Input: part model. Units: mm. Frame: model coordinates. A direction names the side the tool comes from. Coordinates: 2 decimals unless noted, no trailing zeros. Write each loop counter-clockwise with the first axis right and the second up, starting at its lowest first coordinate (ties: lowest second). Pieces come first, ordered by that corner, then holes. Notation, with made-up numbers: M 25.25,-28 L 34.25,-28 A30 ccw 34.25,0 Z; hole C -37.75,0 d8. An arc over 180 degrees is marked long. Use one line per item in the form item = value.
from build123d import *

# Parameters (mm, degrees)
SKETCH1_W               = 117.85
SKETCH1_H               = 100
BOSS_EXTRUDE1_DEPTH     = 3
BOSS_EXTRUDE2_DEPTH     = 117.85
SKETCH3_W               = 10
SKETCH3_H               = 24
CUT_EXTRUDE1_DEPTH      = 3
CUT_EXTRUDE2_DEPTH      = 129.579245993
CUT_EXTRUDE2_DEPTH_BACK = 129.579245993
SKETCH4_W               = 11.05
SKETCH4_H               = 9
SKETCH4_W_2             = 84.75
SKETCH5_W               = 92.85
SKETCH5_H               = 3
CUT_EXTRUDE3_DEPTH      = 3


with BuildPart() as part:
    # Sketch1 → Boss-Extrude1 (new body)
    with BuildSketch(Plane(origin=(0, 0, 0), x_dir=(1, 0, 0), z_dir=(0, 1, 0))):
        with Locations((58.925, 50)):
            Rectangle(SKETCH1_W, SKETCH1_H)
    extrude(amount=BOSS_EXTRUDE1_DEPTH)

    # Sketch2 → Boss-Extrude2 (add)
    with BuildSketch(Plane(origin=(117.85, 0, 0), x_dir=(0, 0, -1), z_dir=(1, 0, 0))):
        Polygon((4.2, 6), (4.2, 3), (6.5, 3), (6.5, 12), (4.2, 12), align=None)
        Polygon((4.2, 12), (4.2, 6), (1.2, 8.517298894), align=None)
    boss_extrude2 = extrude(amount=-BOSS_EXTRUDE2_DEPTH)

    # Sketch3 → Cut-Extrude1 (cut)
    with BuildSketch(Plane.XZ):
        with Locations((112.85, -56)):
            Rectangle(SKETCH3_W, SKETCH3_H)
    extrude(amount=-CUT_EXTRUDE1_DEPTH, mode=Mode.SUBTRACT)

    # Mirror1: Boss-Extrude2 across plane
    add(boss_extrude2.mirror(Plane.XY.offset(-50)))

    # Sketch4 → Cut-Extrude2 (cut, two sides: drawn at the far end of the back side and taken through both)
    with BuildSketch(Plane.XY.offset(-50).offset(-CUT_EXTRUDE2_DEPTH_BACK)):
        with Locations((5.525, 7.5)):
            Rectangle(SKETCH4_W, SKETCH4_H)
        with Locations((112.325, 7.5)):
            Rectangle(SKETCH4_W, SKETCH4_H)
        with Locations((58.925, 7.5)):
            Rectangle(SKETCH4_W_2, SKETCH4_H)
    extrude(amount=CUT_EXTRUDE2_DEPTH + CUT_EXTRUDE2_DEPTH_BACK, mode=Mode.SUBTRACT)

    # Sketch5 → Cut-Extrude3 (cut)
    with BuildSketch(Plane(origin=(0, 0, 0), x_dir=(-1, 0, 0), z_dir=(0, -1, 0))):
        with Locations((-56.425, 13)):
            Rectangle(SKETCH5_W, SKETCH5_H)
        with Locations((-56.425, 18.08)):
            Rectangle(SKETCH5_W, SKETCH5_H)
        with Locations((-56.425, 23.16)):
            Rectangle(SKETCH5_W, SKETCH5_H)
        with Locations((-56.425, 28.24)):
            Rectangle(SKETCH5_W, SKETCH5_H)
        with Locations((-56.425, 33.32)):
            Rectangle(SKETCH5_W, SKETCH5_H)
        with Locations((-56.425, 38.4)):
            Rectangle(SKETCH5_W, SKETCH5_H)
        with Locations((-56.425, 43.48)):
            Rectangle(SKETCH5_W, SKETCH5_H)
        with Locations((-56.425, 48.56)):
            Rectangle(SKETCH5_W, SKETCH5_H)
        with Locations((-56.425, 53.64)):
            Rectangle(SKETCH5_W, SKETCH5_H)
        with Locations((-56.425, 58.72)):
            Rectangle(SKETCH5_W, SKETCH5_H)
        with Locations((-56.425, 63.8)):
            Rectangle(SKETCH5_W, SKETCH5_H)
        with Locations((-56.425, 68.88)):
            Rectangle(SKETCH5_W, SKETCH5_H)
        with Locations((-56.425, 73.96)):
            Rectangle(SKETCH5_W, SKETCH5_H)
        with Locations((-56.425, 79.04)):
            Rectangle(SKETCH5_W, SKETCH5_H)
        with Locations((-56.425, 84.12)):
            Rectangle(SKETCH5_W, SKETCH5_H)
        with Locations((-56.425, 89.2)):
            Rectangle(SKETCH5_W, SKETCH5_H)
    extrude(amount=-CUT_EXTRUDE3_DEPTH, mode=Mode.SUBTRACT)


solid = part.part
(1) First-contact query: pin 1 Ø2.5 at (y, z) = (7.5, -4.5) entering from -X; pin 2 Ø4 at (x, z) = (76.5, -83) entering from +Y; pin 3 Ø3 at (x, y) = (104.5, 8.5) entering from -Z; pin 4 Ø6 at (x, y) = (21.5, 9.5) entering from +Z. Flat tips, straight axial feed; report the tip coordinate or a pass-through.
Computed:
pin_1 = 11.05
pin_2 = 3
pin_3 = -98.8
pin_4 = through
(2) Section query A-A on z = -38.5. Return the cut outline in (x, y), plus the area to 3 significant figures.
Computed:
outline = M 0,0 L 10,0 L 10,3 L 0,3 Z; M 102.85,0 L 117.85,0 L 117.85,3 L 102.85,3 Z
area = 75.0 mm^2
(3) Pull-direction query (Z, two-part tool) for faces 1 (the flat face through (104, 5, -4.2)), 2 (the flat face through (102.85, 1, -18)), 3 (the flat face through (104.088, 10.234, -97.321)); classes: pulls with the +Z half, pulls with the -Z half, needs draft (parallel to the pull), parting line crosses it, or undercut.
Computed:
face_1 = pulls with the +Z half
face_2 = undercut
face_3 = pulls with the -Z half
(4) Line query: probe 1 along Z at (x, y) = (108, 0.5); probe 2 along Y at (x, z) = (108, -43.5). Output: solid intervals per line, ascending.
Computed:
probe_1 = -100 to -68, -44 to 0
probe_2 = 0 to 3
(5) Section query C-C on x = 66. State how many separate pieces and enclosed holes the cut face has, plus the area to 3 significant figures.
Computed:
separate_pieces = 17
enclosed_holes = 0
area = 156 mm^2
(6) Set-up query: faces 4 (the flat face through (13.838, 10.234, -97.321)), 5 (the flat face through (57, 1, -57.22)), 6 (the flat face through (14, 7, -93.5)). Return all of +Z, -Z, +X, -X, +Y, -Y with unobstructed straight access to the full face (end or side cutting, diameter ignored); none if empty.
Computed:
face_4 = -Z, +X, -X, +Y
face_5 = +Y, -Y
face_6 = +X, -X, +Y
(7) Section query B-B on y = 10.5. Return the cut outline in (x, z), plus the area to 3 significant figures.
Computed:
outline = M 11.05,-97.09 L 16.55,-97.09 L 16.55,-93.5 L 11.05,-93.5 Z; M 11.05,-6.5 L 16.55,-6.5 L 16.55,-2.91 L 11.05,-2.91 Z; M 101.3,-97.09 L 106.8,-97.09 L 106.8,-93.5 L 101.3,-93.5 Z; M 101.3,-6.5 L 106.8,-6.5 L 106.8,-2.91 L 101.3,-2.91 Z
area = 79.0 mm^2
